For this review, take the finished solid that the model builds, in its own axes (mm). A direction names the side the tool comes from. Coordinates: 2 decimals unless noted, no trailing zeros. Write each loop counter-clockwise with the first axis right and the second up, starting at its lowest first coordinate (ties: lowest second). Pieces come first, ordered by that corner, then holes. Notation, with made-up numbers: (36, 11) - (83, 11) arc R24 ccw to (83, 40) - close; hole circle Ø2 at (56, 77.5). An arc over 180 degrees is marked (long way). Write each question's results on one line, items separated by ' | '.
from build123d import *

# Parameters (mm, degrees)
F0_R     = 5
F1_DEPTH = 2


with BuildPart() as f1:
    # F0 (on Front) → F1 (new body)
    with BuildSketch(Plane.XZ):
        with BuildLine():
            ThreePointArc((22.238024, 44.782477), (24.011175, 43.857308), (25.745907, 42.861967))
            Line((25.745907, 42.861967), (35.369586, 60.439977))
            ThreePointArc((35.369586, 60.439977), (35.534871, 61.961453), (34.5759, 63.154173))
            ThreePointArc((34.5759, 63.154173), (33.054424, 63.319458), (31.861703, 62.360486))
            Line((31.861703, 62.360486), (22.238024, 44.782477))
        make_face()
        with BuildLine():
            Line((-35.369586, 60.439977), (-25.745907, 42.861967))
            ThreePointArc((-25.745907, 42.861967), (-24.011175, 43.857308), (-22.238024, 44.782477))
            Line((-22.238024, 44.782477), (-31.861703, 62.360486))
            ThreePointArc((-31.861703, 62.360486), (-33.054424, 63.319458), (-34.5759, 63.154173))
            ThreePointArc((-34.5759, 63.154173), (-35.534871, 61.961453), (-35.369586, 60.439977))
        make_face()
        with BuildLine():
            ThreePointArc((-25.745907, 42.861967), (-43.516062, 24.624222), (-50, 0))
            Line((-50, 0), (50, 0))
            ThreePointArc((50, 0), (43.516062, 24.624222), (25.745907, 42.861967))
            ThreePointArc((25.745907, 42.861967), (24.011175, 43.857308), (22.238024, 44.782477))
            ThreePointArc((22.238024, 44.782477), (0, 50), (-22.238024, 44.782477))
            ThreePointArc((-22.238024, 44.782477), (-24.011175, 43.857308), (-25.745907, 42.861967))
        make_face()
        with Locations((-24.011175, 23)):
            Circle(F0_R, mode=Mode.SUBTRACT)
        with Locations((24.011175, 23)):
            Circle(F0_R, mode=Mode.SUBTRACT)
    extrude(amount=F1_DEPTH)


solid = f1.part
Q1. For faces 5 (the face through (43.7, -1, 24.3)), 6 (the face through (-30.625, -0.986, 51.774)), 7 (the face through (-26.982, -0.986, 53.448)), list the 3-axis set-ups (+Z, -Z, +X, -X, +Y, -Y) from which the entire face can be reached by the end or side of a thin tool; tool diameter is ignored.
Results found:
face 5: +X, +Y, -Y | face 6: -X, +Y, -Y | face 7: +Z, +Y, -Y
Q2. Mouldability with a two-part tool opening along Z and no side actions: class faces 1 (the face through (-1, -2, 25)), 2 (the face through (27.117, -0.986, 53.695)), 3 (the face through (-43.337, -0.986, 24.937)), 4 (the face through (30.49, -0.99, 51.53)) as pulls with the +Z half, pulls with the -Z half, needs draft (parallel to the pull), parting line crosses it, or undercut.
Results found:
face 1: needs draft | face 2: pulls with the +Z half | face 3: undercut | face 4: undercut
Q3. Wall thickness on line 1 along X through (y, z) = (-0.5, 21); line 2 along Z through (x, y) = (1, -1.6); line 3 along X through (y, z) = (-1.6, 22.5): over which ranges is each line inside the solid? List them lowest first. Write a range as from..to.
Results found:
line 1: -45.38..-28.59, -19.43..19.43, 28.59..45.38 | line 2: 0..49.99 | line 3: -44.65..-28.99, -19.04..19.04, 28.99..44.65
Q4. Take a section at B-B on z = 51. State the section outline as (x, y) points, plus the area to 3 significant figures.
Results found:
outline: (-30.2, -2) - (-25.64, -2) - (-25.64, 0) - (-30.2, 0) - close; (25.64, -2) - (30.2, -2) - (30.2, 0) - (25.64, 0) - close | area: 18.2 mm2
Q5. For pin 1 (9 mm diameter, centred on x = -24.01, z = 23, fed in from +Y), flat-tipped, find the tip position at first contact; note if it passes through.
Results found:
pin 1: through
Q6. Take a section at D-D on x = 8.5. State the section outline as (y, z) points, plus the area to 3 significant figures.
Results found:
outline: (-2, 0) - (0, 0) - (0, 49.27) - (-2, 49.27) - close | area: 98.5 mm2
Q7. Take a section at A-A on y = -0.3. State the section outline as (x, z) points, plus the area to 3 significant figures.
Results found:
outline: (-50, 0) - (50, 0) arc R50 ccw to (25.75, 42.86) - (35.37, 60.44) arc R2 ccw to (34.58, 63.15) arc R2 ccw to (31.86, 62.36) - (22.24, 44.78) arc R50 ccw to (-22.24, 44.78) - (-31.86, 62.36) arc R2 ccw to (-34.58, 63.15) arc R2 ccw to (-35.37, 60.44) - (-25.75, 42.86) arc R50 ccw to start; hole circle Ø10 at (-24.01, 23); hole circle Ø10 at (24.01, 23) | area: 3,940 mm2
Q8. Take a section at C-C on z = 23. State the section outline as (x, y) points.
Results found:
outline: (-44.4, -2) - (-29.01, -2) - (-29.01, 0) - (-44.4, 0) - close; (-19.01, -2) - (19.01, -2) - (19.01, 0) - (-19.01, 0) - close; (29.01, -2) - (44.4, -2) - (44.4, 0) - (29.01, 0) - close
